Geometry: see drawing. Coordinates: mm, zero at the bounding-box minimum. Coordinates: 2 decimals unless noted, no trailing zeros. Loops run counter-clockwise (first coordinate to the right, second up) from the corner with the lowest first, then second, coordinate; pieces in that order, holes last. Notation, with made-up numbers: (-8.75, 4) -> (37.25, 4) arc R20 ccw to (37.25, 38) -> close; hole circle Ø3 at (-26.5, 43). An arc over 180 degrees is marked (long way). Answer as a JSON object with one key per item and string values.
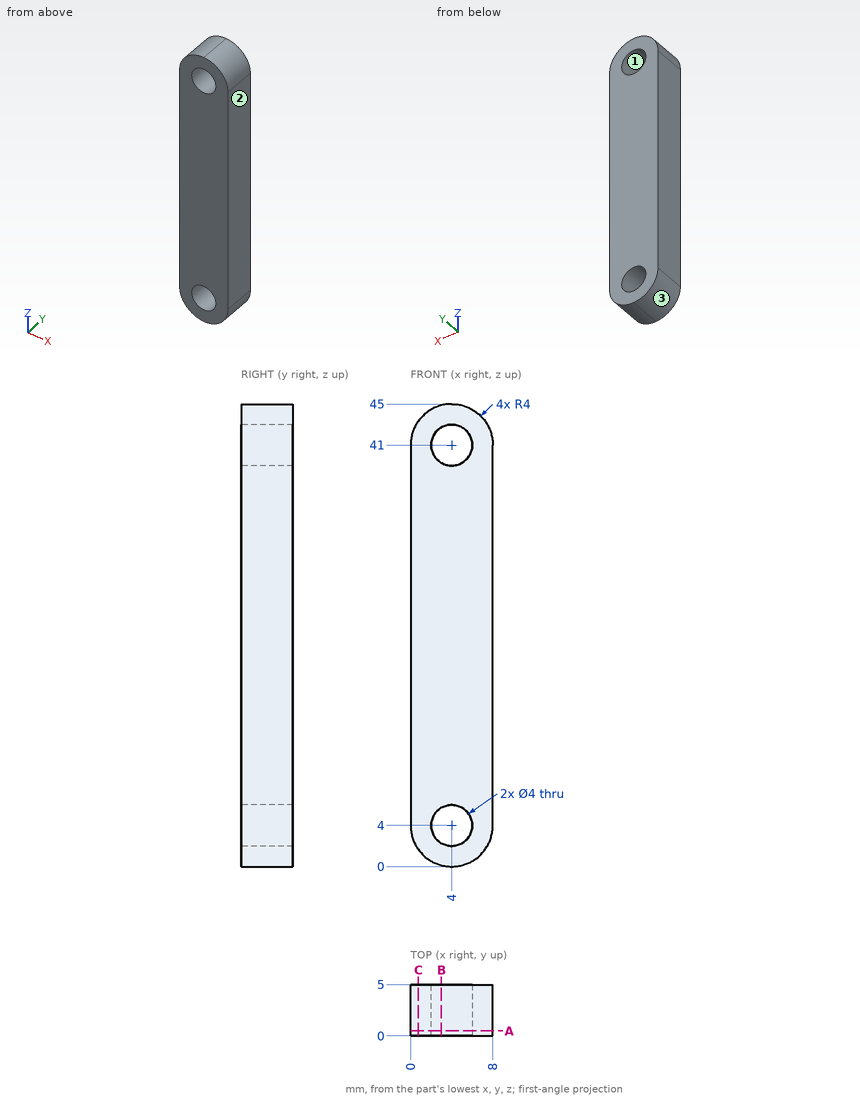
1. Line query: line 1 along Z through (x, y) = (4, 2.4); line 2 along Z through (x, y) = (5.25, 2); line 3 along X through (y, z) = (1.6, 40). Output: solid intervals per line, ascending.
Reply:
{"line 1": "z = 0 to 2, 6 to 39, 43 to 45", "line 2": "z = 0.2 to 2.44, 5.56 to 39.44, 42.56 to 44.8", "line 3": "x = 0 to 2.27, 5.73 to 8"}
2. Section query B-B (x = 3). Return loops of the section in (y, z).
Reply:
{"outline": "(0, 0.13) -> (5, 0.13) -> (5, 2.27) -> (0, 2.27) -> close; (0, 5.73) -> (5, 5.73) -> (5, 39.27) -> (0, 39.27) -> close; (0, 42.73) -> (5, 42.73) -> (5, 44.87) -> (0, 44.87) -> close"}
3. Section query A-A (y = 0.5). Count the separate pieces of the cut face and the enclosed holes in it, plus the area to 3 significant figures.
Reply:
{"separate pieces": "1", "enclosed holes": "2", "area": "321 mm2"}
4. Section query C-C (x = 0.75). Return loops of the section in (y, z), plus the area to 3 significant figures.
Reply:
{"outline": "(0, 1.67) -> (5, 1.67) -> (5, 43.33) -> (0, 43.33) -> close", "area": "208 mm2"}
5. Mould query, pull axis Z, two halves, no side actions, for the marked faces 1, 2 and 3. Classes: pulls with the +Z half, pulls with the -Z half, needs draft (parallel to the pull), parting line crosses it, or undercut.
Reply:
{"face 1": "undercut", "face 2": "needs draft", "face 3": "pulls with the -Z half"}
